```python
from build123d import *

# Parameters (mm, degrees)
SKETCH3_W = 0.254
SKETCH3_H = 0.508


with BuildPart() as part:
    # Sketch1 → Revolve1 (revolve)
    with BuildSketch(Plane.XY):
        Polygon((0, 0), (0, 3.175), (53.1876, 3.175), (53.1876, 9.62025), (74.6506, 9.62025), (74.6506, 0), align=None)
    revolve(axis=Axis((74.6506, 0, 0), (-1, 0, 0)))

    # Sketch2 → Revolve2 (revolve)
    with BuildSketch(Plane.XY):
        Polygon((-12.7, 0), (-12.7, 2.63398), (-12.15898, 3.175), (0, 3.175), (0, 0), align=None)
    revolve(axis=Axis((0, 0, 0), (-1, 0, 0)))

    # Sketch3 → Cut-Revolve1 (revolve, cut)
    with BuildSketch(Plane.XY):
        with Locations((-0.127, 3.175)):
            Rectangle(SKETCH3_W, SKETCH3_H)
    revolve(axis=Axis((0, 0, 0), (-1, 0, 0)), mode=Mode.SUBTRACT)


solid = part.part
```
For this review, take the finished solid that the model builds, in its own axes (mm). A direction names the side the tool comes from. Round coordinates to 2 decimals unless told otherwise and drop trailing zeros. Write each loop counter-clockwise with the first axis right and the second up, starting at its lowest first coordinate (ties: lowest second). Pieces come first, ordered by that corner, then holes. Notation, with made-up numbers: (33, -9) - (63, -9) arc R8 cw to (63, 2) - close; hole circle Ø10 at (45, -22). An arc over 180 degrees is marked (long way). Put each result on its own line as item: value.
Q1. Insertion check: pin 1 Ø1 at (y, z) = (-1.5, -3.5) entering from -X; pin 2 Ø8 at (x, y) = (28.5, -5) entering from +Z; pin 3 Ø3 at (x, y) = (40.5, -3) entering from -Z; pin 4 Ø5 at (x, y) = (55.5, 2.5) entering from -Z. Each pin has a flat end and moves straight along its axis. Give the tip position at first contact, or say it passes through.
Solved:
pin 1: stops at x = 53.19
pin 2: stops at z = 3.01
pin 3: stops at z = -2.8
pin 4: stops at z = -9.62
Q2. We need section C-C (x = 26). Give the boundary of the cut face in (y, z) (3 decimals), and give its area (3 significant figures).
Solved:
outline: circle Ø6.35 at (0, 0)
area: 31.7 mm2
Q3. We need section D-D (x = 67). Give the boundary of the cut face in (y, z), and give its area (3 significant figures).
Solved:
outline: circle Ø19.24 at (0, 0)
area: 291 mm2
Q4. We need section A-A (z = 0). Give the boundary of the cut face in (x, y) (3 decimals).
Solved:
outline: (-12.7, -2.634) - (-12.159, -3.175) - (-0.254, -3.175) - (-0.254, -2.921) - (0, -2.921) - (0, -3.175) - (53.188, -3.175) - (53.188, -9.62) - (74.651, -9.62) - (74.651, 9.62) - (53.188, 9.62) - (53.188, 3.175) - (0, 3.175) - (0, 2.921) - (-0.254, 2.921) - (-0.254, 3.175) - (-12.159, 3.175) - (-12.7, 2.634) - close
Q5. Machinability: for faces 1 (the face through (-12.7, 0, 0)), 2 (the face through (-6.12, -0.69, 3.1)), which of the approach directions +Z, -Z, +X, -X, +Y, -Y give a long, thin tool a straight path to every point of the face, cutting with its end or side? Answer none if there is none.
Solved:
face 1: +Z, -Z, -X, +Y, -Y
face 2: -X
Q6. Wall thickness on probe 1 along X at (y, z) = (2.5, 9); probe 2 along X at (y, z) = (-3, 0.75); probe 3 along Z at (x, y) = (35, 1.75): over which ranges is each line inside the solid? List them lowest first.
Solved:
probe 1: x = 53.19 to 74.65
probe 2: x = -12.24 to -0.25, 0 to 74.65
probe 3: z = -2.65 to 2.65
